The listing builds one solid part. Answer for the finished solid, in the listing's coordinates (mm). Face numbers are marked on the shaded views. Coordinates: 2 decimals unless noted, no trailing zeros. Write each loop counter-clockwise with the first axis right and the second up, starting at its lowest first coordinate (ties: lowest second). Pieces come first, ordered by that corner, then holes.
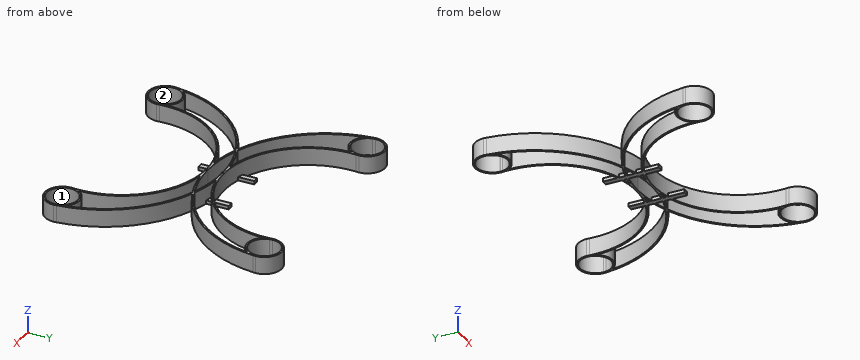
from build123d import *

# Parameters (mm, degrees)
F0_R     = 4.45
F1_DEPTH = 5
F2_W     = 1.6
F2_H     = 16
F3_DEPTH = 1


with BuildPart() as f1:
    # F0 (on Top) → F1 (new body)
    with BuildSketch(Plane.XY):
        with BuildLine():
            ThreePointArc((-12.1246449961, 0.267831512), (-26.0947437129, 10.4656664971), (-33.1275013965, 26.2675592921))
            ThreePointArc((-33.1275013965, 26.2675592921), (-28.7977769223, 24.0541324495), (-24.6632048151, 26.6136413673))
            ThreePointArc((-24.6632048151, 26.6136413673), (-18.7098814469, 10.5941393251), (-3.7729248553, 2.2902948789))
            ThreePointArc((-3.7729248553, 2.2902948789), (-1.8893740867, 2.4475332935), (5.87e-08, 2.5))
            ThreePointArc((5.87e-08, 2.5), (-17.6234951757, 10.132214329), (-24.1138632932, 28.2074294465))
            ThreePointArc((-24.1138632932, 28.2074294465), (-24.0851920036, 28.6039774344), (-24.05, 29))
            ThreePointArc((-24.05, 29), (-29, 33.95), (-33.95, 29))
            ThreePointArc((-33.95, 29), (-33.914900783, 28.5686280089), (-33.8743207345, 28.1377370604))
            ThreePointArc((-33.8743207345, 28.1377370604), (-27.2521637698, 11.1393838049), (-12.8053265827, 0))
            ThreePointArc((-12.8053265827, 0), (-12.4657051208, 0.1357439041), (-12.1246449961, 0.267831512))
        make_face()
        with BuildLine():
            ThreePointArc((-24.6112307284, 28.2643341244), (-28.9708151416, 24.5500957039), (-33.3787423598, 28.206832082))
            ThreePointArc((-33.3787423598, 28.206832082), (-33.4329586461, 28.6109272024), (-33.4499624194, 29.0182883979))
            ThreePointArc((-33.4499624194, 29.0182883979), (-29.0025886323, 33.4499992471), (-24.5500618695, 29.0234656056))
            ThreePointArc((-24.5500618695, 29.0234656056), (-24.5500154674, 29.0117328436), (-24.55, 29))
            ThreePointArc((-24.55, 29), (-24.5653341017, 28.6308951766), (-24.6112307284, 28.2643341244))
        make_face(mode=Mode.SUBTRACT)
        with BuildLine():
            ThreePointArc((-11.4096937343, 0), (-11.7679313517, 0.131881704), (-12.1246449961, 0.267831512))
            ThreePointArc((-12.1246449961, 0.267831512), (-12.4657051208, 0.1357439041), (-12.8053265827, 0))
            ThreePointArc((-12.8053265827, 0), (-12.4657051208, -0.1357439041), (-12.1246449961, -0.267831512))
            ThreePointArc((-12.1246449961, -0.267831512), (-11.7679313517, -0.131881704), (-11.4096937343, 0))
        make_face()
        with BuildLine():
            ThreePointArc((5.87e-08, 2.5), (-1.8893740867, 2.4475332935), (-3.7729248553, 2.2902948789))
            ThreePointArc((-3.7729248553, 2.2902948789), (-1.8920380566, 2.0726808069), (1.392e-07, 2))
            ThreePointArc((1.392e-07, 2), (1.8920381954, 2.0726808176), (3.7729248553, 2.2902948789))
            ThreePointArc((3.7729248553, 2.2902948789), (1.8893741454, 2.4475332902), (5.87e-08, 2.5))
        make_face()
        with BuildLine():
            ThreePointArc((-12.1246449961, -0.267831512), (-12.4657051208, -0.1357439041), (-12.8053265827, 0))
            ThreePointArc((-12.8053265827, 0), (-27.2521637698, -11.1393838049), (-33.8743207345, -28.1377370604))
            ThreePointArc((-33.8743207345, -28.1377370604), (-33.914900783, -28.5686280089), (-33.95, -29))
            ThreePointArc((-33.95, -29), (-29, -33.95), (-24.05, -29))
            ThreePointArc((-24.05, -29), (-24.0851920036, -28.6039774344), (-24.1138632932, -28.2074294465))
            ThreePointArc((-24.1138632932, -28.2074294465), (-17.6234951757, -10.132214329), (5.87e-08, -2.5))
            ThreePointArc((5.87e-08, -2.5), (-1.8893740867, -2.4475332935), (-3.7729248553, -2.2902948789))
            ThreePointArc((-3.7729248553, -2.2902948789), (-18.7098814469, -10.5941393251), (-24.6632048151, -26.6136413673))
            ThreePointArc((-24.6632048151, -26.6136413673), (-28.7977769223, -24.0541324495), (-33.1275013965, -26.2675592921))
            ThreePointArc((-33.1275013965, -26.2675592921), (-26.0947437129, -10.4656664971), (-12.1246449961, -0.267831512))
        make_face()
        with Locations((-29, -29)):
            Circle(F0_R, mode=Mode.SUBTRACT)
        with BuildLine():
            ThreePointArc((24.1138632932, 28.2074294465), (17.6234952159, 10.1322143718), (5.87e-08, 2.5))
            ThreePointArc((5.87e-08, 2.5), (1.8893741454, 2.4475332902), (3.7729248553, 2.2902948789))
            ThreePointArc((3.7729248553, 2.2902948789), (18.7098814469, 10.5941393251), (24.6632048151, 26.6136413673))
            ThreePointArc((24.6632048151, 26.6136413673), (28.7977769223, 24.0541324495), (33.1275013965, 26.2675592921))
            ThreePointArc((33.1275013965, 26.2675592921), (26.0947437129, 10.4656664971), (12.1246449961, 0.267831512))
            ThreePointArc((12.1246449961, 0.267831512), (12.4657051208, 0.1357439041), (12.8053265827, 0))
            ThreePointArc((12.8053265827, 0), (27.2521637698, 11.1393838049), (33.8743207345, 28.1377370604))
            ThreePointArc((33.8743207345, 28.1377370604), (33.914900783, 28.5686280089), (33.95, 29))
            ThreePointArc((33.95, 29), (29, 33.95), (24.05, 29))
            ThreePointArc((24.05, 29), (24.0851920036, 28.6039774344), (24.1138632932, 28.2074294465))
        make_face()
        with BuildLine():
            ThreePointArc((33.3787423598, 28.206832082), (28.9708151416, 24.5500957039), (24.6112307284, 28.2643341244))
            ThreePointArc((24.6112307284, 28.2643341244), (24.5643763362, 28.6425888733), (24.5500618695, 29.0234656056))
            ThreePointArc((24.5500618695, 29.0234656056), (29.0025886323, 33.4499992471), (33.4499624194, 29.0182883979))
            ThreePointArc((33.4499624194, 29.0182883979), (33.4499906049, 29.0091442183), (33.45, 29))
            ThreePointArc((33.45, 29), (33.4321497888, 28.6018188235), (33.3787423598, 28.206832082))
        make_face(mode=Mode.SUBTRACT)
        with BuildLine():
            ThreePointArc((3.7729248553, -2.2902948789), (1.8920381954, -2.0726808176), (1.392e-07, -2))
            ThreePointArc((1.392e-07, -2), (-1.8920380566, -2.0726808069), (-3.7729248553, -2.2902948789))
            ThreePointArc((-3.7729248553, -2.2902948789), (-1.8893740867, -2.4475332935), (5.87e-08, -2.5))
            ThreePointArc((5.87e-08, -2.5), (1.8893741454, -2.4475332902), (3.7729248553, -2.2902948789))
        make_face()
        with BuildLine():
            ThreePointArc((-33.95, 29), (-33.9310438872, 28.5672111577), (-33.8743207345, 28.1377370604))
            ThreePointArc((-33.8743207345, 28.1377370604), (-33.914900783, 28.5686280089), (-33.95, 29))
        make_face()
        with BuildLine():
            ThreePointArc((-33.95, -29), (-33.914900783, -28.5686280089), (-33.8743207345, -28.1377370604))
            ThreePointArc((-33.8743207345, -28.1377370604), (-33.9310438872, -28.5672111577), (-33.95, -29))
        make_face()
        with BuildLine():
            ThreePointArc((12.1246449961, 0.267831512), (11.7679313517, 0.131881704), (11.4096937343, 0))
            ThreePointArc((11.4096937343, 0), (11.7679313517, -0.131881704), (12.1246449961, -0.267831512))
            ThreePointArc((12.1246449961, -0.267831512), (12.4657051208, -0.1357439041), (12.8053265827, 0))
            ThreePointArc((12.8053265827, 0), (12.4657051208, 0.1357439041), (12.1246449961, 0.267831512))
        make_face()
        with BuildLine():
            ThreePointArc((-24.05, 29), (-24.0851920036, 28.6039774344), (-24.1138632932, 28.2074294465))
            ThreePointArc((-24.1138632932, 28.2074294465), (-24.0659916549, 28.6024303198), (-24.05, 29))
        make_face()
        with BuildLine():
            ThreePointArc((24.05, 29), (24.0659916549, 28.6024303198), (24.1138632932, 28.2074294465))
            ThreePointArc((24.1138632932, 28.2074294465), (24.0851920036, 28.6039774344), (24.05, 29))
        make_face()
        with BuildLine():
            ThreePointArc((24.6632048151, -26.6136413673), (18.7098814469, -10.5941393251), (3.7729248553, -2.2902948789))
            ThreePointArc((3.7729248553, -2.2902948789), (1.8893741454, -2.4475332902), (5.87e-08, -2.5))
            ThreePointArc((5.87e-08, -2.5), (17.6234952159, -10.1322143718), (24.1138632932, -28.2074294465))
            ThreePointArc((24.1138632932, -28.2074294465), (24.0851920036, -28.6039774344), (24.05, -29))
            ThreePointArc((24.05, -29), (29, -33.95), (33.95, -29))
            ThreePointArc((33.95, -29), (33.914900783, -28.5686280089), (33.8743207345, -28.1377370604))
            ThreePointArc((33.8743207345, -28.1377370604), (27.2521637698, -11.1393838049), (12.8053265827, 0))
            ThreePointArc((12.8053265827, 0), (12.4657051208, -0.1357439041), (12.1246449961, -0.267831512))
            ThreePointArc((12.1246449961, -0.267831512), (26.0947437129, -10.4656664971), (33.1275013965, -26.2675592921))
            ThreePointArc((33.1275013965, -26.2675592921), (28.7977769223, -24.0541324495), (24.6632048151, -26.6136413673))
        make_face()
        with Locations((29, -29)):
            Circle(F0_R, mode=Mode.SUBTRACT)
        with BuildLine():
            ThreePointArc((-24.1138632932, -28.2074294465), (-24.0851920036, -28.6039774344), (-24.05, -29))
            ThreePointArc((-24.05, -29), (-24.0659916549, -28.6024303198), (-24.1138632932, -28.2074294465))
        make_face()
        with BuildLine():
            ThreePointArc((33.8743207345, 28.1377370604), (33.9310438872, 28.5672111577), (33.95, 29))
            ThreePointArc((33.95, 29), (33.914900783, 28.5686280089), (33.8743207345, 28.1377370604))
        make_face()
        with BuildLine():
            ThreePointArc((24.05, -29), (24.0851920036, -28.6039774344), (24.1138632932, -28.2074294465))
            ThreePointArc((24.1138632932, -28.2074294465), (24.0659916549, -28.6024303198), (24.05, -29))
        make_face()
        with BuildLine():
            ThreePointArc((33.95, -29), (33.9310438872, -28.5672111577), (33.8743207345, -28.1377370604))
            ThreePointArc((33.8743207345, -28.1377370604), (33.914900783, -28.5686280089), (33.95, -29))
        make_face()
        with BuildLine():
            ThreePointArc((-3.7729248553, 2.2902948789), (-8.0128503863, 1.5436201739), (-12.1246449961, 0.267831512))
            ThreePointArc((-12.1246449961, 0.267831512), (-11.7679313517, 0.131881704), (-11.4096937343, 0))
            ThreePointArc((-11.4096937343, 0), (-5.7918284664, 1.4962171068), (1.392e-07, 2))
            ThreePointArc((1.392e-07, 2), (-1.8920380566, 2.0726808069), (-3.7729248553, 2.2902948789))
        make_face()
        with BuildLine():
            ThreePointArc((1.392e-07, -2), (-5.7918284664, -1.4962171068), (-11.4096937343, 0))
            ThreePointArc((-11.4096937343, 0), (-11.7679313517, -0.131881704), (-12.1246449961, -0.267831512))
            ThreePointArc((-12.1246449961, -0.267831512), (-8.0128503863, -1.5436201739), (-3.7729248553, -2.2902948789))
            ThreePointArc((-3.7729248553, -2.2902948789), (-1.8920380566, -2.0726808069), (1.392e-07, -2))
        make_face()
        with BuildLine():
            ThreePointArc((11.4096937343, 0), (5.7918286035, -1.4962170827), (1.392e-07, -2))
            ThreePointArc((1.392e-07, -2), (1.8920381954, -2.0726808176), (3.7729248553, -2.2902948789))
            ThreePointArc((3.7729248553, -2.2902948789), (8.0128503863, -1.5436201739), (12.1246449961, -0.267831512))
            ThreePointArc((12.1246449961, -0.267831512), (11.7679313517, -0.131881704), (11.4096937343, 0))
        make_face()
        with BuildLine():
            ThreePointArc((3.7729248553, 2.2902948789), (1.8920381954, 2.0726808176), (1.392e-07, 2))
            ThreePointArc((1.392e-07, 2), (5.7918286035, 1.4962170827), (11.4096937343, 0))
            ThreePointArc((11.4096937343, 0), (11.7679313517, 0.131881704), (12.1246449961, 0.267831512))
            ThreePointArc((12.1246449961, 0.267831512), (8.0128503863, 1.5436201739), (3.7729248553, 2.2902948789))
        make_face()
    extrude(amount=F1_DEPTH)

    # F2 (on Top) → F3 (join)
    with BuildSketch(Plane.XY):
        with Locations((7.2, 0)):
            Rectangle(F2_W, F2_H)
        with Locations((-7.2, 0)):
            Rectangle(F2_W, F2_H)
    extrude(amount=F3_DEPTH)


solid = f1.part
Q1. Given pin 1 (10 mm diameter, centred on x = -29, y = -29, fed in from -Z); pin 2 (3 mm diameter, centred on x = 1.5, z = 1.5, fed in from +Y); pin 3 (1 mm diameter, centred on y = 2.5, z = 0.5, fed in from +X); pin 4 (0.8 mm diameter, centred on y = -6, z = 0.5, fed in from -X), each flat-ended and moving along its own axis, determine where each tip first touches the part or whether it passes through.
Answers below:
pin 1: stops at z = 0
pin 2: stops at y = 2.69
pin 3: stops at x = 18.55
pin 4: stops at x = -22.95
Q2. Find the intervals of material crossed by probe 1 along X at (y, z) = (-15, 3.2); probe 2 along Y at (x, z) = (-29, 2.05); probe 3 along X at (y, z) = (12, 3.5), in increasing order.
Answers below:
probe 1: x = -29.75 to -29.18, -21.73 to -21.16, 21.16 to 21.73, 29.18 to 29.75
probe 2: y = -33.95 to -33.45, -24.55 to -24.05, -14.68 to -13.71, 13.71 to 14.68, 24.05 to 24.55, 33.45 to 33.95
probe 3: x = -27.88 to -27.26, -19.83 to -19.21, 19.21 to 19.83, 27.26 to 27.88
Q3. The part is cut by section A-A, the plane y = -13.5. Write down the section's boundary in (x, z), then the cut area to 3 significant figures.
Answers below:
outline: (-28.87, 0) - (-28.28, 0) - (-28.28, 5) - (-28.87, 5) - close; (-20.86, 0) - (-20.26, 0) - (-20.26, 5) - (-20.86, 5) - close; (20.26, 0) - (20.86, 0) - (20.86, 5) - (20.26, 5) - close; (28.28, 0) - (28.87, 0) - (28.87, 5) - (28.28, 5) - close
area: 11.9 mm2
Q4. The part is cut by section B-B, the plane x = 10.5. Write down the section's boundary in (y, z), then the cut area to 3 significant figures.
Answers below:
outline: (-4.9, 0) - (-4.35, 0) - (-4.35, 5) - (-4.9, 5) - close; (-0.84, 0) - (-0.31, 0) - (-0.31, 5) - (-0.84, 5) - close; (0.31, 0) - (0.84, 0) - (0.84, 5) - (0.31, 5) - close; (4.35, 0) - (4.9, 0) - (4.9, 5) - (4.35, 5) - close
area: 10.8 mm2
Q5. The part is cut by section D-D, the plane x = -29. Write down the section's boundary in (y, z).
Answers below:
outline: (-33.95, 0) - (-33.45, 0) - (-33.45, 5) - (-33.95, 5) - close; (-24.55, 0) - (-24.05, 0) - (-24.05, 5) - (-24.55, 5) - close; (-14.68, 0) - (-13.71, 0) - (-13.71, 5) - (-14.68, 5) - close; (13.71, 0) - (14.68, 0) - (14.68, 5) - (13.71, 5) - close; (24.05, 0) - (24.55, 0) - (24.55, 5) - (24.05, 5) - close; (33.45, 0) - (33.95, 0) - (33.95, 5) - (33.45, 5) - close
Q6. The part is cut by section C-C, the plane z = 2. State how many separate pieces and enclosed holes the cut face has, then the cut area to 3 significant figures.
Answers below:
separate pieces: 1
enclosed holes: 9
area: 228 mm2
Q7. Determine the mould class of the marked faces 1 and 2 for opening direction X: released by +X, released by -X, zero draft, split by the parting line, or undercut.
Answers below:
face 1: undercut
face 2: undercut
